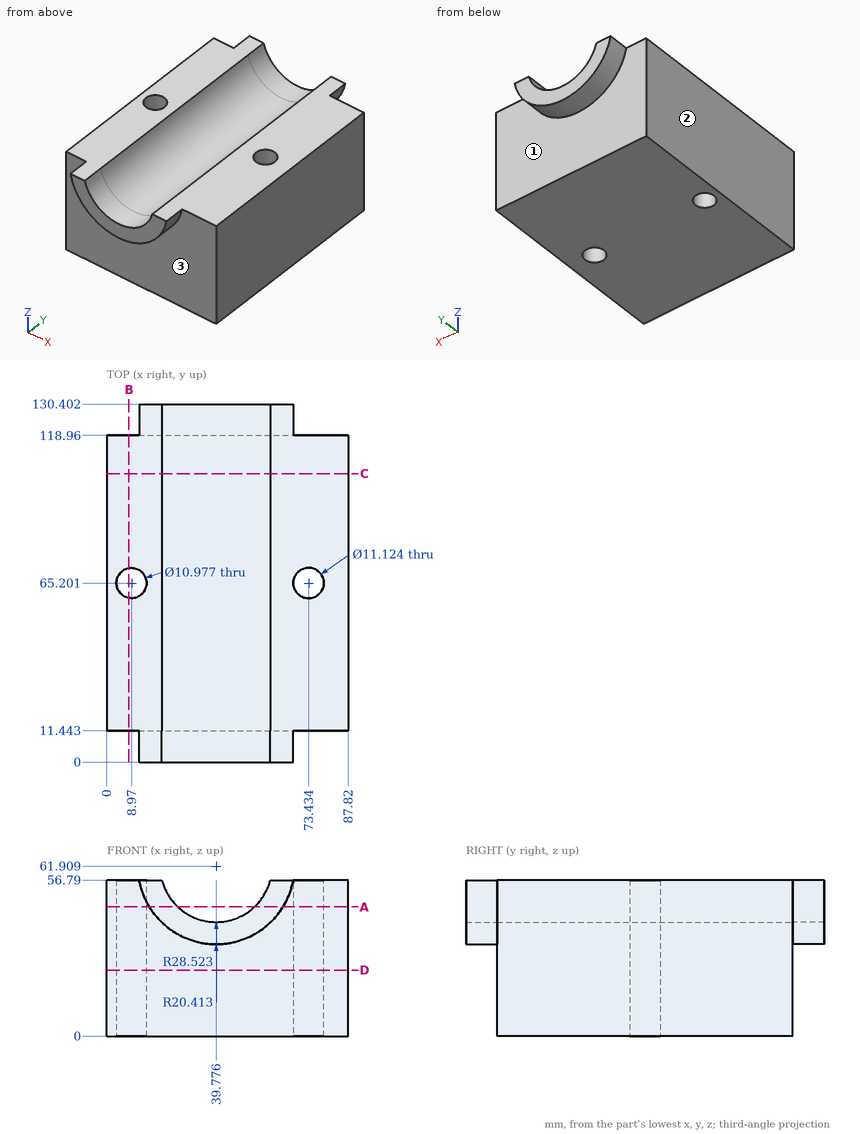
Input: dimensioned drawing with shaded views. Units: mm. Origin: part minimum x, y, z. A direction names the side the tool comes from. Give positions to 0.01 mm unless a question says otherwise; leave off trailing zeros. Loops run counter-clockwise (first coordinate to the right, second up) from the corner with the lowest first, then second, coordinate; pieces in that order, holes last. Notation, with made-up numbers: (31.25, 10) -> (65.25, 10) arc R20 cw to (65.25, 21) -> close; hole circle Ø4 at (-5, 67.5). An arc over 180 degrees is marked (long way). Use a Markdown table: item, result.
Q1. First-contact query: P1, Ø3, axis at x = 33.5, z = 15, coming from the +Y side; P2, Ø3, axis at x = 44, z = 22, coming from the -Y side. Flat tips, straight axial feed; report the tip coordinate or a pass-through.
Entries:
| item | result |
|---|---|
| P1 | stops at y = 118.96 |
| P2 | stops at y = 11.44 |
Q2. Section query A-A, the plane z = 47. Return the cut outline in (x, y) (1 decimal).
Entries:
| item | result |
|---|---|
| outline | (0, 11.4) -> (15.5, 11.4) -> (15.5, 0) -> (25.8, 0) -> (25.8, 130.4) -> (15.5, 130.4) -> (15.5, 119) -> (0, 119) -> close; (53.7, 0) -> (64.1, 0) -> (64.1, 11.4) -> (87.8, 11.4) -> (87.8, 119) -> (64.1, 119) -> (64.1, 130.4) -> (53.7, 130.4) -> close; hole circle Ø11 at (9, 65.2); hole circle Ø11.1 at (73.4, 65.2) |
Q3. Access query for the marked faces 1, 2 and 3. Directions: +Z, -Z, +X, -X, +Y, -Y. A direction counts if a zero-diameter tool reaches every point of the face in a straight line with its end or side. Return the directions, or none.
Entries:
| item | result |
|---|---|
| face 1 | -Z, +Y |
| face 2 | +Z, -Z, -X, +Y, -Y |
| face 3 | -Z, -Y |
Q4. Section query B-B, the plane x = 8. Return the cut outline in (y, z).
Entries:
| item | result |
|---|---|
| outline | (11.44, 0) -> (59.8, 0) -> (59.8, 56.79) -> (11.44, 56.79) -> close; (70.6, 0) -> (118.96, 0) -> (118.96, 56.79) -> (70.6, 56.79) -> close |
Q5. Section query D-D, the plane z = 24. Return the cut outline in (x, y) (1 decimal), plus the area to 3 significant figures.
Entries:
| item | result |
|---|---|
| outline | (0, 11.4) -> (87.8, 11.4) -> (87.8, 119) -> (0, 119) -> close; hole circle Ø11 at (9, 65.2); hole circle Ø11.1 at (73.4, 65.2) |
| area | 9,250 mm² |
Q6. Section query C-C, the plane y = 105. Return the cut outline in (x, z) (1 decimal).
Entries:
| item | result |
|---|---|
| outline | (0, 0) -> (87.8, 0) -> (87.8, 56.8) -> (59.5, 56.8) arc R20.4 cw to (20, 56.8) -> (0, 56.8) -> close |
Q7. Ray query, probe 1 along Y at (x, z) = (37, 20.5); probe 2 along Y at (x, z) = (73.5, 37.5); probe 3 along Y at (x, z) = (71, 31). Return the intervals inside material, ascending. Write a range as from..to.
Entries:
| item | result |
|---|---|
| probe 1 | y = 11.44..118.96 |
| probe 2 | y = 11.44..59.64, 70.76..118.96 |
| probe 3 | y = 11.44..60.2, 70.2..118.96 |
